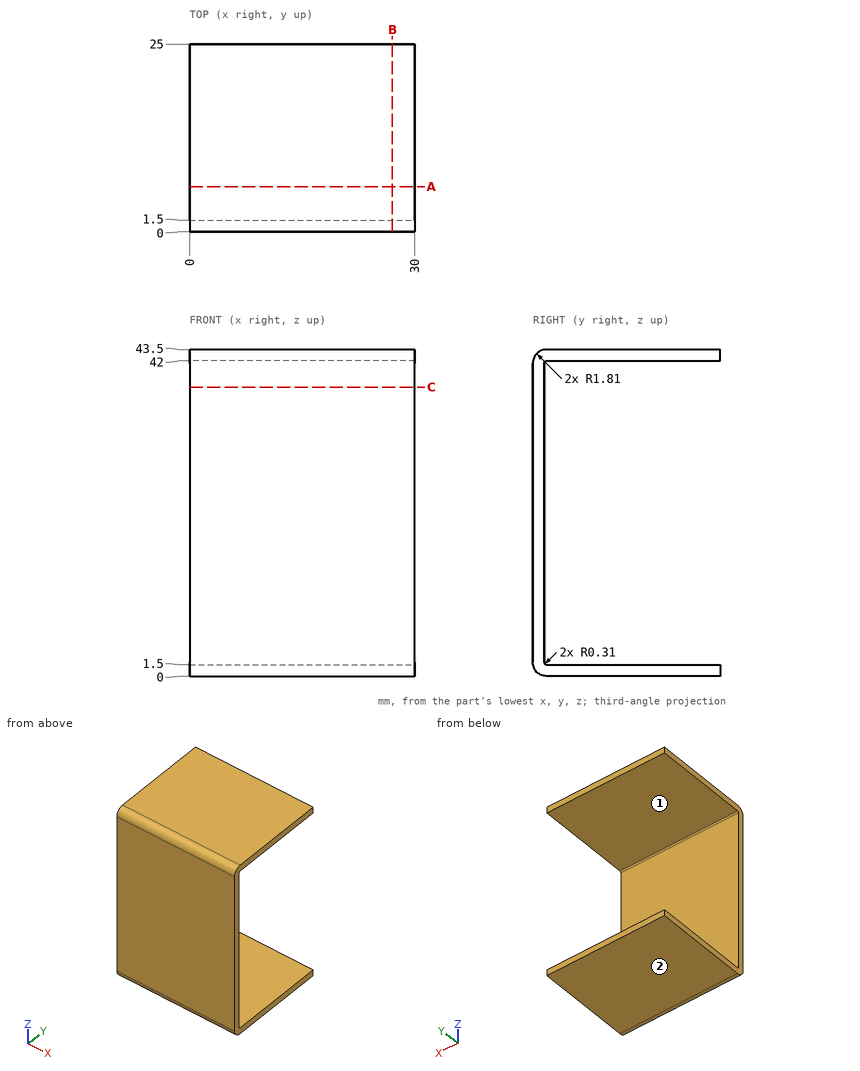
The drawing under review shows one solid part. Ordinate dimensions are in mm from its lowest x, y, z. A direction names the side the tool comes from. Coordinates: 2 decimals unless noted, no trailing zeros. Write each loop counter-clockwise with the first axis right and the second up, starting at its lowest first coordinate (ties: lowest second). Pieces come first, ordered by that corner, then holes.
1) Insertion check: pin 1 (3 mm diameter, centred on x = 14, z = 31, fed in from +Y); pin 2 (8 mm diameter, centred on y = 21, z = 8.5, fed in from +X). Each pin has a flat end and moves straight along its axis. Give the tip position at first contact, or say it passes through.
2) Machinability: for the marked faces 1 and 2, which of the approach directions +Z, -Z, +X, -X, +Y, -Y give a long, thin tool a straight path to every point of the face, cutting with its end or side? Answer none if there is none.
3) Add section A-A (y = 6). Write out the cut boundary in (x, z).
4) To check wall thickness, follow L1, parallel to Z at x = 23, y = 14.75; L2, parallel to Y at x = 19.75, z = 38.5. State the ranges of each line that lie inside material, in increasing order.
5) Add section B-B (x = 27). Write out the cut boundary in (y, z), plus the area to 3 significant figures.
6) Add section C-C (z = 38.5). Write out the cut boundary in (x, y), plus the area to 3 significant figures.
Check result:
1. pin 1: stops at y = 1.5
1. pin 2: passes through
2. face 1: +X, -X, +Y
2. face 2: -Z, +X, -X, +Y, -Y
3. outline: (0, 0) - (30, 0) - (30, 1.5) - (0, 1.5) - close; (0, 42) - (30, 42) - (30, 43.5) - (0, 43.5) - close
4. L1: z = 0 to 1.5, 42 to 43.5
4. L2: y = 0 to 1.5
5. outline: (0, 1.81) arc R1.81 ccw to (1.81, 0) - (25, 0) - (25, 1.5) - (1.81, 1.5) arc R0.31 cw to (1.5, 1.81) - (1.5, 41.69) arc R0.31 cw to (1.81, 42) - (25, 42) - (25, 43.5) - (1.81, 43.5) arc R1.81 ccw to (0, 41.69) - close
5. area: 134 mm2
6. outline: (0, 0) - (30, 0) - (30, 1.5) - (0, 1.5) - close
6. area: 45.0 mm2
